Read the model definition and answer for the solid it produces. Units are mm, in the model's axes. A direction names the side the tool comes from. Round coordinates to 2 decimals unless told otherwise and drop trailing zeros. Write each loop counter-clockwise with the first axis right and the second up, starting at its lowest first coordinate (ties: lowest second). Pieces come first, ordered by that corner, then holes. Notation, with made-up numbers: (-9.5, -33.5) - (49.5, -33.5) arc R6 ccw to (49.5, -23.5) - close; hole circle Ø1 at (47.5, 74.5). An arc over 180 degrees is marked (long way). Use one line per item in the form item = value. Start each with the question number.
1) The part is cut by section D-D, the plane x = 37. Give the vertices of the cut face in (y, z), plus the area to 3 significant figures.
2) The part is cut by section B-B, the plane z = 46.5. Give the vertices of the cut face in (x, y).
3) The part is cut by section A-A, the plane y = 76. Give the vertices of the cut face in (x, z), plus the area to 3 significant figures.
4) Each of these flat-tipped pins is pushed along its axis until it touches: pin 1 (2 mm diameter, centred on y = 100.5, z = -54.5, fed in from +X); pin 2 (25 mm diameter, centred on x = 41, y = 54.5, fed in from -Z); pin 3 (16 mm diameter, centred on y = 77.5, z = 55.5, fed in from -X). Where does it stop, or does it pass through?
5) The part is cut by section C-C, the plane x = 20.5. Give the vertices of the cut face in (y, z), plus the area to 3 significant figures.
6) For faces 1 (the face through (-21.492, 69, 49)), 2 (the face through (21, 49, 64.422)), 3 (the face through (62.334, 70, -48)), 4 (the face through (20, 49, 32.5)), determine the directions among +Z, -Z, +X, -X, +Y, -Y from which every point of the face is accessible in a straight line to the end or side of a thin tool.
7) For a pull along Z with two mould halves and no side action, classify faces 5 (the face through (62.334, 70, 49)), 6 (the face through (20, 49, -32.5)), 7 (the face through (21, 49, -64.422)), 8 (the face through (19, 107.442, 0)) as released by +Z, released by -Z, zero draft, split by the parting line, or undercut.
8) Consider line 1 along Z through (x, y) = (48, 28.5); line 2 along Y through (x, z) = (-0.5, -27); line 3 along X through (y, z) = (42.5, 61.5). Determine where each line is inside the solid, lowest interval first. Write a range as from..to.
from build123d import *

# Parameters (mm, degrees)
SKETCH4_R           = 5
BOSS_EXTRUDE4_DEPTH = 64.422352731
SKETCH6_W           = 94.412285725
SKETCH6_H           = 145.116249754
BOSS_EXTRUDE5_DEPTH = 16.844705461
SKETCH7_W           = 105.313643584
SKETCH7_H           = 127.479897163
CUT_EXTRUDE1_DEPTH  = 32.5


with BuildPart() as part:
    # Sketch4 → Boss-Extrude4 (new body, symmetric)
    with BuildSketch(Plane.XY):
        with BuildLine():
            Line((-21.492390891, 31.428545296), (-21.492390891, 107.442049888))
            Line((-21.492390891, 107.442049888), (62.333666954, 107.442049888))
            Line((62.333666954, 107.442049888), (62.333666954, 31.428545296))
            ThreePointArc((62.333666954, 31.428545296), (20.420638031, -10.484483627), (-21.492390891, 31.428545296))
        make_face()
        with Locations((20.420638031, 31.428545296)):
            Circle(SKETCH4_R, mode=Mode.SUBTRACT)
    extrude(amount=BOSS_EXTRUDE4_DEPTH, both=True)

    # Sketch6 → Boss-Extrude5 (add)
    with BuildSketch(Plane(origin=(0, 107.442049888, 0), x_dir=(1, 0, 0), z_dir=(0, 1, 0))):
        with Locations((20.027144796, -0.604818135)):
            Rectangle(SKETCH6_W, SKETCH6_H)
    extrude(amount=BOSS_EXTRUDE5_DEPTH)

    # Sketch7 → Cut-Extrude1 (cut, symmetric)
    with BuildSketch(Plane.XY):
        with Locations((20.29997807, 43.702101306)):
            Rectangle(SKETCH7_W, SKETCH7_H)
    extrude(amount=CUT_EXTRUDE1_DEPTH, both=True, mode=Mode.SUBTRACT)


solid = part.part
Geometry results:
q1.outline = (-7.07, -64.42) - (107.44, -64.42) - (107.44, -71.95) - (124.29, -71.95) - (124.29, 73.16) - (107.44, 73.16) - (107.44, 64.42) - (-7.07, 64.42) - (-7.07, 32.5) - (107.44, 32.5) - (107.44, -32.5) - (-7.07, -32.5) - close
q1.area = 9,760 mm2
q2.outline = (-27.18, 107.44) - (-21.49, 107.44) - (-21.49, 31.43) arc R41.91 ccw to (62.33, 31.43) - (62.33, 107.44) - (67.23, 107.44) - (67.23, 124.29) - (-27.18, 124.29) - close; hole circle Ø10 at (20.42, 31.43)
q3.outline = (-21.49, -64.42) - (62.33, -64.42) - (62.33, -32.5) - (-21.49, -32.5) - close; (-21.49, 32.5) - (62.33, 32.5) - (62.33, 64.42) - (-21.49, 64.42) - close
q3.area = 5,350 mm2
q4.pin_1 = 62.33
q4.pin_2 = -64.42
q4.pin_3 = -21.49
q5.outline = (-10.48, -64.42) - (26.43, -64.42) - (26.43, -32.5) - (-10.48, -32.5) - close; (-10.48, 32.5) - (26.43, 32.5) - (26.43, 64.42) - (-10.48, 64.42) - close; (36.43, -64.42) - (107.44, -64.42) - (107.44, -71.95) - (124.29, -71.95) - (124.29, 73.16) - (107.44, 73.16) - (107.44, 64.42) - (36.43, 64.42) - (36.43, 32.5) - (107.44, 32.5) - (107.44, -32.5) - (36.43, -32.5) - close
q5.area = 9,340 mm2
q6.face_1 = +Z, -Z, -X, -Y
q6.face_2 = +Z, +X, -X, -Y
q6.face_3 = +Z, -Z, +X, -Y
q6.face_4 = +X, -X, -Y
q7.face_5 = zero draft
q7.face_6 = undercut
q7.face_7 = released by -Z
q7.face_8 = undercut
q8.line_1 = -64.42..-32.5, 32.5..64.42
q8.line_2 = 107.44..124.29
q8.line_3 = -21.49..62.33
